from build123d import *

# Parameters (mm, degrees)
F0_R     = 30
F1_DEPTH = 25
F2_W     = 20
F2_H     = 10
F3_DEPTH = 39.7
F4_R     = 4
F5_DEPTH = 41.2
F7_D     = 5


with BuildPart() as f1:
    # F0 (on Top) → F1 (new body)
    with BuildSketch(Plane.XY):
        Circle(F0_R)
    extrude(amount=F1_DEPTH)

    # F2 (on face) → F3 (join)
    with BuildSketch(Plane.XY.offset(25)):
        with Locations((0.236175, -5)):
            Rectangle(F2_W, F2_H)
    extrude(amount=F3_DEPTH)

    # F4 (on face) → F5 (cut)
    with BuildSketch(Plane(origin=(0, 0, 0), x_dir=(-1, 0, 0), z_dir=(0, 1, 0))):
        with Locations((0, 55.906373)):
            Circle(F4_R)
    extrude(amount=-F5_DEPTH, mode=Mode.SUBTRACT)

    # F7 (through all)
    with Locations(Plane.XZ.offset(10)):
        with Locations((0, 40.813621)):
            Hole(F7_D / 2)


solid = f1.part
For this review, take the finished solid that the model builds, in its own axes (mm). A direction names the side the tool comes from. Give positions to 0.01 mm unless a question says otherwise; leave off trailing zeros. Order: outer loops, then holes, each group sorted by start corner. A loop starts at its lowest first (then second) coordinate and runs counter-clockwise, first axis right, second up. Notation, with made-up numbers: M 70.5,17 L 79.5,17 A37 cw 79.5,55 Z; hole C 57,38 d11. An arc over 180 degrees is marked long. Answer in a Markdown table with one row per item. Add a question column.
(1) Mouldability with a two-part tool opening along Z and no side actions: class faces 5 (the face through (-29.97, 1.32, 12.32)), 6 (the face through (0.521, -4.93, 59.872)), 7 (the face through (-1.344, -4.93, 42.922)), 8 (the face through (0, -5, 64.7)) as +Z half, -Z half, draft (parallel to the pull), parting line (faces both ways), or undercut.
(2) Consider section A-A on x = 0. State the section outline as (y, z) points, and give its area (3 significant figures).
(3) Consider section D-D on y = 6. State the section outline as (x, z) points, and give its area (3 significant figures).
(4) Consider section C-C on x = 6. State the section outline as (y, z) points.
(5) Consider section B-B on z = 8.5. State the section outline as (x, y) points, and give its area (3 significant figures).
(6) Wall thickness on probe 1 along Z at (x, y) = (0, -4); probe 2 along Z at (x, y) = (-24, -17); probe 3 along X at (y, z) = (-6.5, 61.5): over which ranges is each line inside the solid? List them lowest first. Write a range as [from, to].
(7) For faces 1 (the face through (0, 0, 45)), 2 (the face through (-9.764, -5, 45)), 3 (the face through (0, -10, 45)), 4 (the face through (10.236, -5, 45)), list the 3-axis set-ups (+Z, -Z, +X, -X, +Y, -Y) from which the entire face can be reached by the end or side of a thin tool; tool diameter is ignored.
(8) For pin 1 (4 mm diameter, centred on y = -6.5, z = 47, fed in from -X); pin 2 (6.5 mm diameter, centred on x = 0, z = 40.81, fed in from +Y); pin 3 (6 mm diameter, centred on x = -2, z = 50, fed in from -Y), all flat-tipped, find the tip position at first contact; note any pin that passes through.
Evaluation:
| question | item | result |
|---|---|---|
| 1 | face 5 | draft |
| 1 | face 6 | undercut |
| 1 | face 7 | undercut |
| 1 | face 8 | +Z half |
| 2 | outline | M -30,0 L 30,0 L 30,25 L 0,25 L 0,38.31 L -10,38.31 L -10,25 L -30,25 Z; M -10,43.31 L 0,43.31 L 0,51.91 L -10,51.91 Z; M -10,59.91 L 0,59.91 L 0,64.7 L -10,64.7 Z |
| 2 | area | 1,770 mm^2 |
| 3 | outline | M -29.39,0 L 29.39,0 L 29.39,25 L -29.39,25 Z |
| 3 | area | 1,470 mm^2 |
| 4 | outline | M -29.39,0 L 29.39,0 L 29.39,25 L 0,25 L 0,64.7 L -10,64.7 L -10,25 L -29.39,25 Z |
| 5 | outline | C 0,0 d60 |
| 5 | area | 2,830 mm^2 |
| 6 | probe 1 | z = [0, 38.31], [43.31, 51.91], [59.91, 64.7] |
| 6 | probe 2 | z = [0, 25] |
| 6 | probe 3 | x = [-9.76, 10.24] |
| 7 | face 1 | +Z, +X, -X, +Y |
| 7 | face 2 | +Z, -X, +Y, -Y |
| 7 | face 3 | +Z, +X, -X, -Y |
| 7 | face 4 | +Z, +X, +Y, -Y |
| 8 | pin 1 | stops at x = -9.76 |
| 8 | pin 2 | stops at y = 0 |
| 8 | pin 3 | stops at y = -10 |
